from build123d import *

# Parameters (mm, degrees)
SKETCH_1_R      = 1.5
EXTRUDE_1_DEPTH = 1.6
EXTRUDE_START   = 1.6
SKETCH_2_W      = 22.7
SKETCH_2_H      = 7
SKETCH_2_W_2    = 7
SKETCH_2_H_2    = 12.5
EXTRUDE_2_DEPTH = 5.8


with BuildPart() as part:
    # 草图1 → 凸台-拉伸1 (new body)
    with BuildSketch(Plane(origin=(0, 0, 0), x_dir=(1, 0, 0), z_dir=(0, 1, 0))):
        with BuildLine():
            Line((-15.5, -19.5), (15.5, -19.5))
            ThreePointArc((15.5, -19.5), (18.328427125, -18.328427125), (19.5, -15.5))
            Line((19.5, -15.5), (19.5, 15.5))
            ThreePointArc((19.5, 15.5), (18.328427125, 18.328427125), (15.5, 19.5))
            Line((15.5, 19.5), (-15.5, 19.5))
            ThreePointArc((-15.5, 19.5), (-18.328427125, 18.328427125), (-19.5, 15.5))
            Line((-19.5, 15.5), (-19.5, -15.5))
            ThreePointArc((-19.5, -15.5), (-18.328427125, -18.328427125), (-15.5, -19.5))
        make_face()
        with Locations(Location((-15.5, -15.5, 0), (0, 0, 270))):
            Circle(SKETCH_1_R, mode=Mode.SUBTRACT)
        with Locations(Location((15.5, -15.5, 0), (0, 0, 270))):
            Circle(SKETCH_1_R, mode=Mode.SUBTRACT)
        with Locations(Location((-15.5, 15.5, 0), (0, 0, 270))):
            Circle(SKETCH_1_R, mode=Mode.SUBTRACT)
        with Locations(Location((15.5, 15.5, 0), (0, 0, 270))):
            Circle(SKETCH_1_R, mode=Mode.SUBTRACT)
    extrude(amount=EXTRUDE_1_DEPTH)

    # 草图2 → 凸台-拉伸2 (add)
    with BuildSketch(Plane(origin=(0, 0, 0), x_dir=(1, 0, 0), z_dir=(0, 1, 0)).offset(EXTRUDE_START)):
        with Locations((0, 19.7)):
            Rectangle(SKETCH_2_W, SKETCH_2_H)
        with Locations((-21, 0)):
            Rectangle(SKETCH_2_W_2, SKETCH_2_H_2)
    extrude(amount=EXTRUDE_2_DEPTH)


solid = part.part
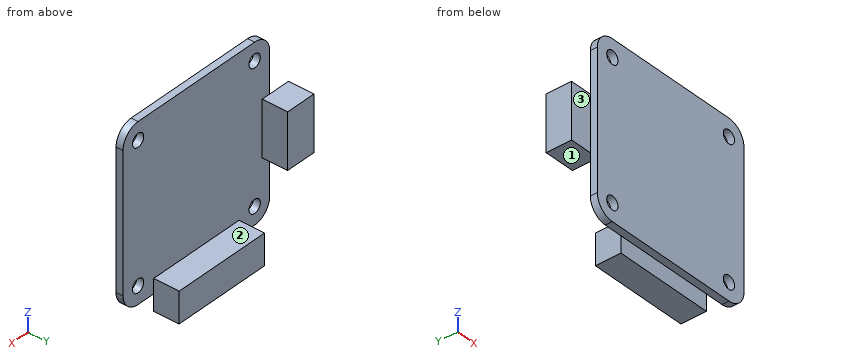
Part model, mm, in its own coordinate system. Face numbers are marked on the shaded views. A direction names the side the tool comes from. Coordinates: 2 decimals unless noted, no trailing zeros. Order: outer loops, then holes, each group sorted by start corner. A loop starts at its lowest first (then second) coordinate and runs counter-clockwise, first axis right, second up. Notation, with made-up numbers: M 27.25,46.5 L 44.25,46.5 A12 cw 44.25,66.5 Z; hole C 20,62.5 d7. An arc over 180 degrees is marked long. One line per question, with ' | ' between items.
Q1. Slice it at A-A (y = 3.5). Give the cut face in (x, z), and give its area (3 significant figures).
A:
outline: M -24.5,-6.25 L -17.5,-6.25 L -17.5,6.25 L -24.5,6.25 Z; M -11.35,-23.2 L 11.35,-23.2 L 11.35,-16.2 L -11.35,-16.2 Z | area: 246 mm^2
Q2. 3-axis set-ups, long thin cutter, end or side, ignore diameter. For the marked faces 1, 2 and 3: which of +Z, -Z, +X, -X, +Y, -Y reach the whole face in a straight line?
A:
face 1: -Z, +X, -X, +Y | face 2: +Z, +X, -X, +Y | face 3: +Z, -Z, -X, -Y
Q3. Drill centre lines: line 1 (X direction, y = 0.8, z = -15.5); line 2 (Y direction, x = -4, z = 4); line 3 (Z direction, x = -8, y = 2.5). Where is each one in solid material? Low to high.
A:
line 1: x = -19.5 to -17, -14 to 14, 17 to 19.5 | line 2: y = 0 to 1.6 | line 3: z = -23.2 to -16.2
Q4. Slice it at B-B (x = -1). Give the cut face in (y, z).
A:
outline: M 0,-19.5 L 1.6,-19.5 L 1.6,-23.2 L 7.4,-23.2 L 7.4,-16.2 L 1.6,-16.2 L 1.6,19.5 L 0,19.5 Z
Q5. Slice it at D-D (z = -1.5). Give the cut face in (x, y), and give its area (3 significant figures).
A:
outline: M -24.5,1.6 L -19.5,1.6 L -19.5,0 L 19.5,0 L 19.5,1.6 L -17.5,1.6 L -17.5,7.4 L -24.5,7.4 Z | area: 103 mm^2
Q6. Slice it at C-C (y = 1). Give the cut face in (x, z), and give its area (3 significant figures).
A:
outline: M -19.5,-15.5 A4 ccw -15.5,-19.5 L 15.5,-19.5 A4 ccw 19.5,-15.5 L 19.5,15.5 A4 ccw 15.5,19.5 L -15.5,19.5 A4 ccw -19.5,15.5 Z; hole C -15.5,-15.5 d3; hole C -15.5,15.5 d3; hole C 15.5,-15.5 d3; hole C 15.5,15.5 d3 | area: 1,480 mm^2
Q7. Pin check, flat tips, straight feed: P1, Ø5, axis at x = -15.5, z = 15.5, coming from the +Y side; P2, Ø0.5, axis at y = 0.5, z = 1, coming from the -X side; P3, Ø1.7, axis at x = -22.5, y = 6, coming from the -Z side. Stop position of each tip, or through.
A:
P1: stops at y = 1.6 | P2: stops at x = -19.5 | P3: stops at z = -6.25
